Design review of the part built by this model. Coordinates are the model's own, in mm. A direction names the side the tool comes from. Coordinates: 2 decimals unless noted, no trailing zeros. Write each loop counter-clockwise with the first axis right and the second up, starting at its lowest first coordinate (ties: lowest second). Pieces come first, ordered by that corner, then holes. Notation, with made-up numbers: M 69.25,34.25 L 75.25,34.25 A20 ccw 75.25,65.25 Z; hole C -22,-27.5 d7. An arc over 180 degrees is marked long. One line per question, with ' | ' between items.
from build123d import *

# Parameters (mm, degrees)
F0_R     = 35
F0_R_2   = 27
F1_DEPTH = 20
F2_START = 15
F2_DEPTH = 5
F3_R     = 8.25
F3_R_2   = 4
F4_DEPTH = 100
F5_DEPTH = 12


with BuildPart() as f1:
    # F0 (on Top) → F1 (new body)
    with BuildSketch(Plane.XY):
        Circle(F0_R)
        Circle(F0_R_2, mode=Mode.SUBTRACT)
    extrude(amount=F1_DEPTH)

    # F0 (on Top) → F2 (join)
    with BuildSketch(Plane.XY.offset(F2_START)):
        Circle(F0_R_2)
    extrude(amount=F2_DEPTH)

    # F3 (on face) → F4 (join)
    with BuildSketch(Plane.XY.offset(20)):
        Circle(F3_R)
        Circle(F3_R_2, mode=Mode.SUBTRACT)
    extrude(amount=F4_DEPTH)

    # F5 (cut): a face of the model
    f5_faces = [f1.faces().sort_by_distance(p)[0] for p in [
        (0, 0, 20),
    ]]
    extrude(f5_faces, amount=-F5_DEPTH, mode=Mode.SUBTRACT)


solid = f1.part
1. Draft analysis for pull direction X (two halves, no side actions). For faces 1 (the face through (7, -7, 20)), 2 (the face through (-5.85, -26.36, 7.4)), 3 (the face through (7.62, -3.16, 69.3)), state which applies: pulls with the +X half, pulls with the -X half, needs draft (parallel to the pull), parting line crosses it, or undercut.
Answer sheet:
face 1: needs draft | face 2: undercut | face 3: parting line crosses it
2. Tool access review of faces 4 (the face through (-2, -4, 120)), 5 (the face through (6, 0, 15)): name each direction out of +Z, -Z, +X, -X, +Y, -Y from which nothing blocks a thin tool from reaching the whole face with its end or side.
Answer sheet:
face 4: +Z, +X, -X, +Y, -Y | face 5: -Z
3. To check wall thickness, follow line 1 along Y through (x, z) = (0, 11); line 2 along Y through (x, z) = (0, 16); line 3 along Z through (x, y) = (17, 30.5). State the ranges of each line that lie inside material, in increasing order. Write a range as [from, to].
Answer sheet:
line 1: [-35, -27], [27, 35] | line 2: [-35, -4], [4, 35] | line 3: [0, 20]
4. Take a section at D-D (x = 25.5). Write out the cut boundary in (y, z).
Answer sheet:
outline: M -23.97,0 L -8.87,0 L -8.87,15 L 8.87,15 L 8.87,0 L 23.97,0 L 23.97,20 L -23.97,20 Z
5. Take a section at A-A (y = 0). Write out the cut boundary in (x, z).
Answer sheet:
outline: M -35,0 L -27,0 L -27,15 L -4,15 L -4,120 L -8.25,120 L -8.25,20 L -35,20 Z; M 4,15 L 27,15 L 27,0 L 35,0 L 35,20 L 8.25,20 L 8.25,120 L 4,120 Z
6. Insertion check: pin 1 Ø4 at (x, y) = (24.5, 19) entering from +Z; pin 2 Ø13 at (x, y) = (0, 0) entering from -Z; pin 3 Ø5 at (x, z) = (-17, 13.5) entering from +Y; pin 4 Ø12 at (x, y) = (12, -26.5) entering from -Z. Each pin has a flat end and moves straight along its axis. Give the tip position at first contact, or say it passes through.
Answer sheet:
pin 1: z = 20 | pin 2: z = 15 | pin 3: y = 31.86 | pin 4: z = 0
7. Take a section at C-C (z = 108). Write out the cut boundary in (x, y), then the cut area to 3 significant figures.
Answer sheet:
outline: C 0,0 d16.5; hole C 0,0 d8 | area: 164 mm^2
